```python
from build123d import *

# Parameters (mm, degrees)
SKETCH1_W           = 50
SKETCH1_H           = 25.4
SKETCH1_R           = 1.725
SKETCH1_H_2         = 25
BOSS_EXTRUDE1_DEPTH = 3.175
FILLET1_R           = 2


with BuildPart() as part:
    # Sketch1 → Boss-Extrude1 (new body)
    # profile 1 of 2: a face of its own
    with BuildSketch(Plane(origin=(0, 0, 0), x_dir=(1, 0, 0), z_dir=(0, 1, 0))):
        with Locations((22.5, -2.7)):
            Rectangle(SKETCH1_W, SKETCH1_H)
        with Locations(Location((0, 0, 0), (0, 0, 270))):
            Circle(SKETCH1_R, mode=Mode.SUBTRACT)
        with Locations(Location((45, 0, 0), (0, 0, 270))):
            Circle(SKETCH1_R, mode=Mode.SUBTRACT)
    # profile 2 of 2: a face of its own
    with BuildSketch(Plane(origin=(0, 0, 0), x_dir=(1, 0, 0), z_dir=(0, 1, 0))):
        with Locations((22.5, -27.9)):
            Rectangle(SKETCH1_W, SKETCH1_H_2)
    extrude(amount=BOSS_EXTRUDE1_DEPTH)

    # Fillet1
    fillet1_edges = [part.edges().sort_by_distance(p)[0] for p in [
        (47.5, 1.5875, 40.4),
        (-2.5, 1.5875, 40.4),
        (-2.5, 1.5875, -10),
        (47.5, 1.5875, -10),
    ]]
    fillet(fillet1_edges, radius=FILLET1_R)


solid = part.part
```
Geometry: final body of the model. Coordinates: model frame, mm. Coordinates: 2 decimals unless noted, no trailing zeros. Order: outer loops, then holes, each group sorted by start corner. A loop starts at its lowest first (then second) coordinate and runs counter-clockwise, first axis right, second up. Notation, with made-up numbers: (54.5, 10.5) - (92.5, 10.5) arc R26 ccw to (92.5, 46.5) - close; hole circle Ø3 at (33.5, 53). An arc over 180 degrees is marked (long way). Return JSON: item names as keys, results as strings. Group by question number.
1. Cut plane A-A (z = 0). Output: boundary loops of the cut face in (x, y) (3 decimals).
2. Material intervals for line 1 along X through (y, z) = (2, 0) (3 decimals), sorted ascending. Write a range as [from, to].
3. Pull-direction query (Z, two-part tool) for faces 1 (the face through (43.316, 1.565, -0.374)), 2 (the face through (-1.93, 1.61, 39.8)), 3 (the face through (22, 2, -10)); classes: pulls with the +Z half, pulls with the -Z half, needs draft (parallel to the pull), parting line crosses it, or undercut.
4. Pin query (flat end, axial travel): pin 1 (10 mm diameter, centred on x = 5.5, z = 11.5, fed in from -Y). Return the tip coordinate at first contact, or that it passes through.
Resolved:
{
 "1": {"outline": "(-2.5, 0) - (-1.725, 0) - (-1.725, 3.175) - (-2.5, 3.175) - close; (1.725, 0) - (43.275, 0) - (43.275, 3.175) - (1.725, 3.175) - close; (46.725, 0) - (47.5, 0) - (47.5, 3.175) - (46.725, 3.175) - close"},
 "2": {"line 1": "x = [-2.5, -1.725], [1.725, 43.275], [46.725, 47.5]"},
 "3": {"face 1": "undercut", "face 2": "pulls with the +Z half", "face 3": "pulls with the -Z half"},
 "4": {"pin 1": "stops at y = 0"}
}
